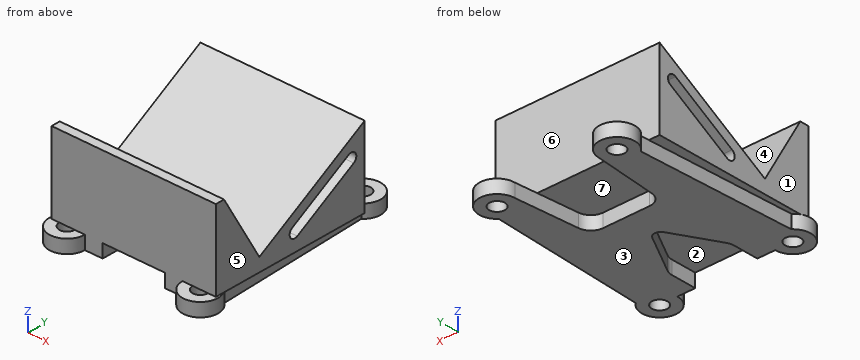
from build123d import *

# Parameters (mm, degrees)
F0_R     = 1.75
F1_DEPTH = 3
F3_DEPTH = 18.5


with BuildPart() as f1:
    # F0 (on Top) → F1 (new body)
    with BuildSketch(Plane.XY):
        with BuildLine():
            ThreePointArc((16, 17.627501), (15.232051, 24.355551), (9.5, 20.75))
            Line((9.5, 20.75), (8.24144, 6.486319))
            ThreePointArc((8.24144, 6.486319), (7.279001, 4.537417), (5.25305, 3.75))
            Line((5.25305, 3.75), (0, 3.75))
            Line((0, 3.75), (-5.25305, 3.75))
            ThreePointArc((-5.25305, 3.75), (-7.279001, 4.537417), (-8.24144, 6.486319))
            Line((-8.24144, 6.486319), (-9.5, 20.75))
            ThreePointArc((-9.5, 20.75), (-15.232051, 24.355551), (-16, 17.627501))
            Line((-16, 17.627501), (-17.5, -17.627501))
            ThreePointArc((-17.5, -17.627501), (-16.732051, -24.355551), (-11, -20.75))
            Line((-11, -20.75), (-7, -20.75))
            Line((-7, -20.75), (-7, -15.028129))
            ThreePointArc((-7, -15.028129), (-6.903908, -14.274924), (-6.621788, -13.56997))
            Line((-6.621788, -13.56997), (-1.310894, -4.02092))
            ThreePointArc((-1.310894, -4.02092), (0, -3.25), (1.310894, -4.02092))
            Line((1.310894, -4.02092), (6.621788, -13.56997))
            ThreePointArc((6.621788, -13.56997), (6.903908, -14.274924), (7, -15.028129))
            Line((7, -15.028129), (7, -20.75))
            Line((7, -20.75), (11, -20.75))
            ThreePointArc((11, -20.75), (16.732051, -24.355551), (17.5, -17.627501))
            Line((17.5, -17.627501), (16, 17.627501))
        make_face()
        with Locations((-15, -20.75)):
            Circle(F0_R, mode=Mode.SUBTRACT)
        with Locations((15, -20.75)):
            Circle(F0_R, mode=Mode.SUBTRACT)
        with Locations((-13.5, 20.75)):
            Circle(F0_R, mode=Mode.SUBTRACT)
        with Locations((13.5, 20.75)):
            Circle(F0_R, mode=Mode.SUBTRACT)
    extrude(amount=F1_DEPTH)

    # F2 (on Right) → F3 (join, symmetric)
    with BuildSketch(Plane.YZ):
        Polygon((-20.75, 21), (-20.75, 3), (15.75, 3), (15.75, 20.918584), (-10.089746, 6), (-18.75, 21), align=None)
        with BuildLine():
            Line((-2.036543, 8.051443), (11.819864, 16.051443))
            ThreePointArc((11.819864, 16.051443), (13.527395, 15.593911), (13.069864, 13.886379))
            Line((13.069864, 13.886379), (-0.786543, 5.886379))
            ThreePointArc((-0.786543, 5.886379), (-2.494074, 6.343911), (-2.036543, 8.051443))
        make_face(mode=Mode.SUBTRACT)
    extrude(amount=F3_DEPTH, both=True)


solid = f1.part
Input: part model. Units: mm. Frame: model coordinates. Face numbers are marked on the shaded views. A direction names the side the tool comes from. Coordinates: 2 decimals unless noted, no trailing zeros. Order: outer loops, then holes, each group sorted by start corner. A loop starts at its lowest first (then second) coordinate and runs counter-clockwise, first axis right, second up.
1. Draft query along X for the marked faces 5, 6 and 7. Return one class per face: +X half, -X half, draft (parallel to the pull), parting line (faces both ways), or undercut.
Checked values:
face 5: +X half
face 6: draft
face 7: undercut
2. Cut plane B-B, the plane y = 3. Return loops of the section in (x, z).
Checked values:
outline: (-18.5, 3) - (-16.62, 3) - (-16.62, 0) - (16.62, 0) - (16.62, 3) - (18.5, 3) - (18.5, 8.07) - (-18.5, 8.07) - close; (-18.5, 10.96) - (18.5, 10.96) - (18.5, 13.56) - (-18.5, 13.56) - close
3. Cut plane A-A, the plane z = 10.75. Return loops of the section in (x, y).
Checked values:
outline: (-18.5, -20.75) - (18.5, -20.75) - (18.5, -12.83) - (-18.5, -12.83) - close; (-18.5, -1.86) - (18.5, -1.86) - (18.5, 2.64) - (-18.5, 2.64) - close; (-18.5, 7.64) - (18.5, 7.64) - (18.5, 15.75) - (-18.5, 15.75) - close
4. Ray query, line 1 along Y through (x, z) = (-15, 1.55); line 2 along Y through (x, z) = (13.5, 0.7); line 3 along X through (y, z) = (-17, 3.5). Return the intervals inside material, ascending.
Checked values:
line 1: y = -24.75 to -22.5, -19 to 19.85, 21.65 to 24.46
line 2: y = -24.46 to -21.65, -19.85 to 19, 22.5 to 24.75
line 3: x = -18.5 to 18.5
5. Access query for the marked faces 1, 2, 3 and 4. Directions: +Z, -Z, +X, -X, +Y, -Y. A direction counts if a zero-diameter tool reaches every point of the face in a straight line with its end or side. Return the directions, or none.
Checked values:
face 1: +Z, -X, +Y, -Y
face 2: -Z, -Y
face 3: -Z, +X, -X, +Y, -Y
face 4: +Z, +X, -X
6. Cut plane D-D, the plane z = 15.25. Return loops of the section in (x, y).
Checked values:
outline: (-18.5, -20.75) - (18.5, -20.75) - (18.5, -15.43) - (-18.5, -15.43) - close; (-18.5, 5.93) - (18.5, 5.93) - (18.5, 10.43) - (-18.5, 10.43) - close; (-18.5, 13.66) - (18.5, 13.66) - (18.5, 15.75) - (-18.5, 15.75) - close
7. Contact query for flat-ended pins moving along their axis: P1, Ø3, axis at x = 5, y = -6, coming from the +Z side; P2, Ø12, axis at x = 1.5, z = 15.5, coming from the -Y side; P3, Ø4, axis at x = -12, y = 4, coming from the +Z side. Output: stop coordinate, or through.
Checked values:
P1: stops at z = 9.23
P2: stops at y = -20.75
P3: stops at z = 15.29
8. Cut plane C-C, the plane x = -6. Return loops of the section in (y, z), plus the area to 3 significant figures.
Checked values:
outline: (-20.75, 3) - (-12.45, 3) - (-12.45, 0) - (3.84, 0) - (3.84, 3) - (15.75, 3) - (15.75, 20.92) - (-10.09, 6) - (-18.75, 21) - (-20.75, 21) - close; hole (-2.04, 8.05) arc R1.25 ccw to (-0.79, 5.89) - (13.07, 13.89) arc R1.25 ccw to (11.82, 16.05) - close
area: 401 mm2
